Source: CAD feature listing. Evaluate the final solid. Frame: model axes, mm. Coordinates: 2 decimals unless noted, no trailing zeros. Loops run counter-clockwise (first coordinate to the right, second up) from the corner with the lowest first, then second, coordinate; pieces in that order, holes last.
from build123d import *

# Parameters (mm, degrees)
SKETCH2_R           = 5
SKETCH2_W           = 120
SKETCH2_H           = 120
BOSS_EXTRUDE1_DEPTH = 10
SKETCH3_R           = 2.5
CUT_EXTRUDE1_DEPTH  = 10


with BuildPart() as part:
    # Sketch2 → Boss-Extrude1 (new body)
    with BuildSketch(Plane.XY):
        with BuildLine():
            Line((-75, 90), (75, 90))
            ThreePointArc((75, 90), (85.606601718, 85.606601718), (90, 75))
            Line((90, 75), (90, -75))
            ThreePointArc((90, -75), (85.606601718, -85.606601718), (75, -90))
            Line((75, -90), (-75, -90))
            ThreePointArc((-75, -90), (-85.606601718, -85.606601718), (-90, -75))
            Line((-90, -75), (-90, 75))
            ThreePointArc((-90, 75), (-85.606601718, 85.606601718), (-75, 90))
        make_face()
        with Locations((-75, 75)):
            Circle(SKETCH2_R, mode=Mode.SUBTRACT)
        with Locations((0, 75)):
            Circle(SKETCH2_R, mode=Mode.SUBTRACT)
        with Locations((75, 75)):
            Circle(SKETCH2_R, mode=Mode.SUBTRACT)
        with Locations((-75, 0)):
            Circle(SKETCH2_R, mode=Mode.SUBTRACT)
        with Locations((75, 0)):
            Circle(SKETCH2_R, mode=Mode.SUBTRACT)
        with Locations((-75, -75)):
            Circle(SKETCH2_R, mode=Mode.SUBTRACT)
        with Locations((0, -75)):
            Circle(SKETCH2_R, mode=Mode.SUBTRACT)
        with Locations((75, -75)):
            Circle(SKETCH2_R, mode=Mode.SUBTRACT)
        Rectangle(SKETCH2_W, SKETCH2_H, mode=Mode.SUBTRACT)
    extrude(amount=BOSS_EXTRUDE1_DEPTH)

    # Sketch3 → Cut-Extrude1 (cut)
    with BuildSketch(Plane.XY.offset(10)):
        with Locations((-60, 60)):
            Circle(SKETCH3_R)
        with Locations((60, 60)):
            Circle(SKETCH3_R)
        with Locations((60, -60)):
            Circle(SKETCH3_R)
        with Locations((-60, -60)):
            Circle(SKETCH3_R)
    extrude(amount=-CUT_EXTRUDE1_DEPTH, mode=Mode.SUBTRACT)


solid = part.part
Q1. Section A-A, the plane y = 0. Return the cut outline in (x, z).
Q2. Line query: line 1 along Y through (x, z) = (-52.5, 1.5); line 2 along Y through (x, z) = (-75, 7.5). Output: solid intervals per line, ascending.
Q3. Draft query along X for faces 1 (the flat face through (-90, -1, 5)), 2 (the flat face through (-1, 60, 5)), 3 (the flat face through (1, 61, 10)). Return one class per face: +X half, -X half, draft (parallel to the pull), parting line (faces both ways), or undercut.
Q4. Contact query for a flat-ended pin moving along its axis: pin 1 Ø8 at (x, y) = (0, -75) entering from -Z. Output: stop coordinate, or through.
Q5. Section B-B, the plane y = -46. Return the cut outline in (x, z).
Q6. Section D-D, the plane z = 5. Count the separate pieces of the cut face and the enclosed holes in it, plus the area to 3 significant figures.
Derived:
1. outline: (-90, 0) - (-80, 0) - (-80, 10) - (-90, 10) - close; (-70, 0) - (-60, 0) - (-60, 10) - (-70, 10) - close; (60, 0) - (70, 0) - (70, 10) - (60, 10) - close; (80, 0) - (90, 0) - (90, 10) - (80, 10) - close
2. line 1: y = -90 to -60, 60 to 90
2. line 2: y = -90 to -80, -70 to -5, 5 to 70, 80 to 90
3. face 1: -X half
3. face 2: undercut
3. face 3: draft
4. pin 1: passes through
5. outline: (-90, 0) - (-60, 0) - (-60, 10) - (-90, 10) - close; (60, 0) - (90, 0) - (90, 10) - (60, 10) - close
6. separate pieces: 1
6. enclosed holes: 9
6. area: 17,100 mm2
